Model file for the job. Use its own axes, mm. Face numbers are marked on the shaded views. Coordinates: 2 decimals unless noted, no trailing zeros. Order: outer loops, then holes, each group sorted by start corner. A loop starts at its lowest first (then second) coordinate and runs counter-clockwise, first axis right, second up. Notation, with made-up numbers: (31.25, 22) -> (65.25, 22) arc R32 cw to (65.25, 51) -> close; hole circle Ø1 at (4.5, -14). An arc over 180 degrees is marked (long way). Return JSON: item names as keys, results as strings. Group by question number.
1) Cut at C-C (x = -13.5). Write the cut outline in (y, z).
2) Pull direction X, two halves, no side cores. Call the marked faces 1 and 2: +X half, -X half, draft (parallel to the pull), parting line (faces both ways), or undercut.
3) Flat gauge pins, fed straight in: pin 1 (1.2 mm diameter, centred on x = -33, y = 0, fed in from +Z); pin 2 (2 mm diameter, centred on y = -0.5, z = -67.5, fed in from +X); pin 3 (10 mm diameter, centred on x = -14.5, z = 49, fed in from -Y). Where does each tip first touch, or does it go through?
4) Cut at B-B (z = 11). Write the cut outline in (x, y), and give its area (3 significant figures).
5) Probe line 1 (X direction, y = -1.25, z = -50.5); line 2 (Z direction, x = -21, y = -2.5); line 3 (Y direction, x = -27.5, z = 33.5). List the from-to ranges inside material, lowest first.
6) Cut at D-D (x = -0.5). Write the cut outline in (y, z).
7) Cut at A-A (y = -0.5). Write the cut outline in (x, z), and give its area (3 significant figures).
from build123d import *

# Parameters (mm, degrees)
F0_W      = 67.1
F0_H      = 138.3
F1_DEPTH  = 3.55
F2_R      = 5
F3_T      = -2.5
F5_DEPTH  = 12.5
F6_W      = 17.2149091959
F6_H      = 4.6
F7_DEPTH  = 12.5
F8_W      = 4.6
F8_H      = 25.1665320247
F9_DEPTH  = 12.5
F10_W     = 4.6
F10_H     = 13.3939161897
F11_DEPTH = 12.5


with BuildPart() as f1:
    # F0 (on Front) → F1 (new body, symmetric)
    with BuildSketch(Plane.XZ):
        Rectangle(F0_W, F0_H)
    extrude(amount=F1_DEPTH, both=True)

    # F2
    f2_edges = [f1.edges().sort_by_distance(p)[0] for p in [
        (-33.55, 0, 69.15),
        (33.55, 0, 69.15),
        (-33.55, 0, -69.15),
        (33.55, 0, -69.15),
    ]]
    fillet(f2_edges, radius=F2_R)

    # F3
    f3_openings = [f1.faces().sort_by_distance(p)[0] for p in [
        (0, -3.55, 0),
    ]]
    offset(amount=F3_T, openings=f3_openings)

    # F4 (on Front) → F5 (cut, symmetric)
    with BuildSketch(Plane.XZ):
        with BuildLine():
            add(Edge.make_bspline(
                [(13.5491024703, 63.1798133254), (17.0743458114, 65.6223290722), (29.066168273, 65.8951681057), (30.1492148881, 53.2998867845), (9.159231679, 54.5898814711), (11.1556270119, 61.5214592968), (13.5491024703, 63.1798133254)],
                knots=[0, 0, 0, 0, 0.2904013559, 0.4958031268, 0.8028310527, 1, 1, 1, 1], degree=3))
        make_face()
    extrude(amount=F5_DEPTH, both=True, mode=Mode.SUBTRACT)

    # F6 (on face) → F7 (cut, symmetric)
    with BuildSketch(Plane.XY.offset(-66.65)):
        with Locations((0, -1.25)):
            Rectangle(F6_W, F6_H)
    extrude(amount=F7_DEPTH, both=True, mode=Mode.SUBTRACT)

    # F8 (on face) → F9 (cut, symmetric)
    with BuildSketch(Plane.YZ.offset(-31.05)):
        with Locations((-1.25, 35.5272786692)):
            Rectangle(F8_W, F8_H)
    extrude(amount=F9_DEPTH, both=True, mode=Mode.SUBTRACT)

    # F10 (on face) → F11 (cut, symmetric)
    with BuildSketch(Plane(origin=(31.05, 0, 0), x_dir=(0, -1, 0), z_dir=(-1, 0, 0))):
        with Locations((1.25, 43.2292446494)):
            Rectangle(F10_W, F10_H)
    extrude(amount=F11_DEPTH, both=True, mode=Mode.SUBTRACT)


solid = f1.part
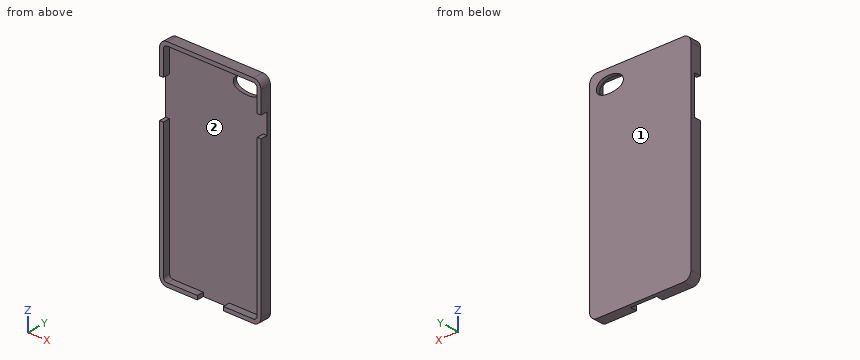
Answers below:
{
 "1": {"outline": "(-3.55, -69.15) -> (3.55, -69.15) -> (3.55, 69.15) -> (-3.55, 69.15) -> (-3.55, 66.65) -> (1.05, 66.65) -> (1.05, -66.65) -> (-3.55, -66.65) -> close"},
 "2": {"face 1": "draft", "face 2": "undercut"},
 "3": {"pin 1": "stops at z = 67.34", "pin 2": "stops at x = 32.96", "pin 3": "stops at y = 1.05"},
 "4": {"outline": "(-33.55, -3.55) -> (-31.05, -3.55) -> (-31.05, 1.05) -> (31.05, 1.05) -> (31.05, -3.55) -> (33.55, -3.55) -> (33.55, 3.55) -> (-33.55, 3.55) -> close", "area": "191 mm^2"},
 "5": {"line 1": "x = -33.55 to -31.05, 31.05 to 33.55", "line 2": "z = -69.15 to -66.65, 66.65 to 69.15", "line 3": "y = 1.05 to 3.55"},
 "6": {"outline": "(-3.55, 66.65) -> (1.05, 66.65) -> (1.05, -69.15) -> (3.55, -69.15) -> (3.55, 69.15) -> (-3.55, 69.15) -> close"},
 "7": {"outline": "(-33.55, -64.15) arc R5 ccw to (-28.55, -69.15) -> (-8.61, -69.15) -> (-8.61, -66.65) -> (-28.55, -66.65) arc R2.5 cw to (-31.05, -64.15) -> (-31.05, 22.94) -> (-33.55, 22.94) -> close; (-33.55, 48.11) -> (-31.05, 48.11) -> (-31.05, 64.15) arc R2.5 cw to (-28.55, 66.65) -> (28.55, 66.65) arc R2.5 cw to (31.05, 64.15) -> (31.05, 49.93) -> (33.55, 49.93) -> (33.55, 64.15) arc R5 ccw to (28.55, 69.15) -> (-28.55, 69.15) arc R5 ccw to (-33.55, 64.15) -> close; (8.61, -69.15) -> (28.55, -69.15) arc R5 ccw to (33.55, -64.15) -> (33.55, 36.53) -> (31.05, 36.53) -> (31.05, -64.15) arc R2.5 cw to (28.55, -66.65) -> (8.61, -66.65) -> close", "area": "846 mm^2"}
}
